The model under review builds one solid part; all positions refer to its coordinate system, in mm. A direction names the side the tool comes from. Coordinates: 2 decimals unless noted, no trailing zeros. Loops run counter-clockwise (first coordinate to the right, second up) from the corner with the lowest first, then second, coordinate; pieces in that order, holes last. Notation, with made-up numbers: M 64,84 L 73,84 A19 ccw 73,95 Z; hole C 76.25,-4.75 d1. An arc over 180 degrees is marked long. Return JSON: item names as keys, results as strings.
```python
from build123d import *

# Parameters (mm, degrees)
BOSS_EXTRUDE1_DEPTH = 3.175
SKETCH2_W           = 9.906
SKETCH2_H           = 9.525
CUT_EXTRUDE1_DEPTH  = 190.835760674
FILLET1_R           = 2.54


with BuildPart() as part:
    # Sketch1 → Boss-Extrude1 (new body)
    with BuildSketch(Plane.XY):
        Polygon((19.05, 0), (-19.05, 0), (-19.05, 7.62), (-128.27, 7.62), (-145.034, 36.656099738), (-95.504, 122.444576237), (-73.506954744, 109.744576237), (-115.704606325, 36.656099738), (-113.605303163, 33.02), (113.605303163, 33.02), (115.704606325, 36.656099738), (73.506954744, 109.744576237), (95.504, 122.444576237), (145.034, 36.656099738), (128.27, 7.62), (19.05, 7.62), align=None)
    extrude(amount=BOSS_EXTRUDE1_DEPTH)

    # Sketch2 → Cut-Extrude1 (cut, through all)
    with BuildSketch(Plane.XY.offset(3.175)):
        with Locations((-79.883, 12.3825)):
            Rectangle(SKETCH2_W, SKETCH2_H)
        Polygon((-112.776, 92.528594689), (-104.527108029, 87.766094689), (-109.480108029, 79.187247039), (-117.729, 83.949747039), align=None)
        Polygon((-73.506954744, 109.744576237), (-102.836348419, 109.744576237), (-95.504, 122.444576237), align=None)
        Polygon((95.504, 122.444576237), (73.506954744, 109.744576237), (102.836348419, 109.744576237), align=None)
        Polygon((117.729, 83.949747039), (112.776, 92.528594689), (104.527108029, 87.766094689), (109.480108029, 79.187247039), align=None)
        with Locations((79.883, 12.3825)):
            Rectangle(SKETCH2_W, SKETCH2_H)
    extrude(amount=-CUT_EXTRUDE1_DEPTH, mode=Mode.SUBTRACT)

    # Fillet1
    fillet1_edges = [part.edges().sort_by_distance(p)[0] for p in [
        (-113.605303163, 33.02, 1.5875),
        (113.605303163, 33.02, 1.5875),
        (115.704606325, 36.656099738, 1.5875),
        (73.506954744, 109.744576237, 1.5875),
        (-73.506954744, 109.744576237, 1.5875),
        (-115.704606325, 36.656099738, 1.5875),
    ]]
    fillet(fillet1_edges, radius=FILLET1_R)


solid = part.part
```
1. Machinability: for faces 1 (the face through (108.71, 90.18, 1.61)), 2 (the face through (-108.71, 90.18, 1.61)), 3 (the face through (106.969, 83.537, 1.61)), which of the approach directions +Z, -Z, +X, -X, +Y, -Y give a long, thin tool a straight path to every point of the face, cutting with its end or side? Answer none if there is none.
Check values:
{"face 1": "+Z, -Z, +X", "face 2": "+Z, -Z, -X", "face 3": "+Z, -Z"}
2. The part is to be moulded in two halves that separate along Y. For faces 4 (the face through (-106.969, 83.537, 1.61)), 5 (the face through (-136.53, 21.93, 1.57)), 6 (the face through (2, 31, 0)), say which applies: released by +Y, released by -Y, zero draft, split by the parting line, or undercut.
Check values:
{"face 4": "undercut", "face 5": "released by -Y", "face 6": "zero draft"}
3. Add section A-A on y = 97. Give the boundary of the cut face in (x, z) (3 decimals), plus the area to 3 significant figures.
Check values:
{"outline": "M -110.194,0 L -80.865,0 L -80.865,3.175 L -110.194,3.175 Z; M 80.865,0 L 110.194,0 L 110.194,3.175 L 80.865,3.175 Z", "area": "186 mm²"}
4. Add section B-B on x = 30.5. Give the boundary of the cut face in (y, z) (3 decimals).
Check values:
{"outline": "M 7.62,0 L 33.02,0 L 33.02,3.175 L 7.62,3.175 Z"}
5. Add section C-C on y = 29. Give the boundary of the cut face in (x, z) (3 decimals).
Check values:
{"outline": "M -140.614,0 L 140.614,0 L 140.614,3.175 L -140.614,3.175 Z"}
6. To check wall thickness, follow line 1 (X direction, y = 17, z = 2.85); line 2 (X direction, y = 9, z = 2); line 3 (X direction, y = 69.5, z = 2.3). State the ranges of each line that lie inside material, in increasing order.
Check values:
{"line 1": "-133.69 to -84.84, -74.93 to 74.93, 84.84 to 133.69", "line 2": "-129.07 to -84.84, -74.93 to 74.93, 84.84 to 129.07", "line 3": "-126.07 to -96.74, 96.74 to 126.07"}
7. Insertion check: pin 1 Ø1 at (y, z) = (10.5, 1) entering from +X; pin 2 Ø1 at (x, y) = (16, 26.5) entering from -Z; pin 3 Ø1 at (x, z) = (-97, 2) entering from -Y; pin 4 Ø1.6 at (x, z) = (80.5, 2) entering from -Y (3 decimals). Each pin has a flat end and moves straight along its axis. Give the tip position at first contact, or say it passes through.
Check values:
{"pin 1": "x = 130.22", "pin 2": "z = 0", "pin 3": "y = 7.62", "pin 4": "y = 17.145"}
